from build123d import *

# Parameters (mm, degrees)
EXTRUDE1_DEPTH = 5.9944


with BuildPart() as part:
    # Sketch1 → Extrude1 (new body)
    with BuildSketch(Plane.XY):
        with BuildLine():
            Line((-209.059629258, -14.077865934), (-209.059629258, -29.477865934))
            Line((-209.059629258, -29.477865934), (58.656370742, -29.477865934))
            Line((58.656370742, -29.477865934), (58.656370742, -14.077865934))
            Line((58.656370742, -14.077865934), (64.650770742, -14.077865934))
            Line((64.650770742, -14.077865934), (64.650770742, -4.077865934))
            Line((64.650770742, -4.077865934), (58.656370742, -4.077865934))
            Line((58.656370742, -4.077865934), (58.656370742, 6.581535434))
            Line((58.656370742, 6.581535434), (49.512370742, 6.581535434))
            Line((49.512370742, 6.581535434), (49.512370742, 4.644785434))
            Line((49.512370742, 4.644785434), (45.512370742, 4.733384066))
            Line((45.512370742, 4.733384066), (45.512370742, 12.670884066))
            Line((45.512370742, 12.670884066), (49.512370742, 12.582285434))
            Line((49.512370742, 12.582285434), (49.512370742, 10.645535434))
            Line((49.512370742, 10.645535434), (58.656370742, 10.645535434))
            Line((58.656370742, 10.645535434), (58.656370742, 21.482134066))
            Line((58.656370742, 21.482134066), (64.650770742, 21.482134066))
            Line((64.650770742, 21.482134066), (64.650770742, 31.482134066))
            Line((64.650770742, 31.482134066), (58.656370742, 31.482134066))
            Line((58.656370742, 31.482134066), (58.656370742, 49.262134066))
            Line((58.656370742, 49.262134066), (27.756302278, 49.262134066))
            ThreePointArc((27.756302278, 49.262134066), (13.878151139, 27.724950493), (0, 49.262134066))
            Line((0, 49.262134066), (-209.059629258, 49.262134066))
            Line((-209.059629258, 49.262134066), (-209.059629258, 31.482134066))
            Line((-209.059629258, 31.482134066), (-215.054029258, 31.482134066))
            Line((-215.054029258, 31.482134066), (-215.054029258, 21.482134066))
            Line((-215.054029258, 21.482134066), (-209.059629258, 21.482134066))
            Line((-209.059629258, 21.482134066), (-209.059629258, 10.822732699))
            Line((-209.059629258, 10.822732699), (-199.915629258, 10.822732699))
            Line((-199.915629258, 10.822732699), (-199.915629258, 12.759482699))
            Line((-199.915629258, 12.759482699), (-195.915629258, 12.670884066))
            Line((-195.915629258, 12.670884066), (-195.915629258, 4.733384066))
            Line((-195.915629258, 4.733384066), (-199.915629258, 4.821982699))
            Line((-199.915629258, 4.821982699), (-199.915629258, 6.758732699))
            Line((-199.915629258, 6.758732699), (-209.059629258, 6.758732699))
            Line((-209.059629258, 6.758732699), (-209.059629258, -4.077865934))
            Line((-209.059629258, -4.077865934), (-215.054029258, -4.077865934))
            Line((-215.054029258, -4.077865934), (-215.054029258, -14.077865934))
            Line((-215.054029258, -14.077865934), (-209.059629258, -14.077865934))
        make_face()
    extrude(amount=EXTRUDE1_DEPTH)


solid = part.part
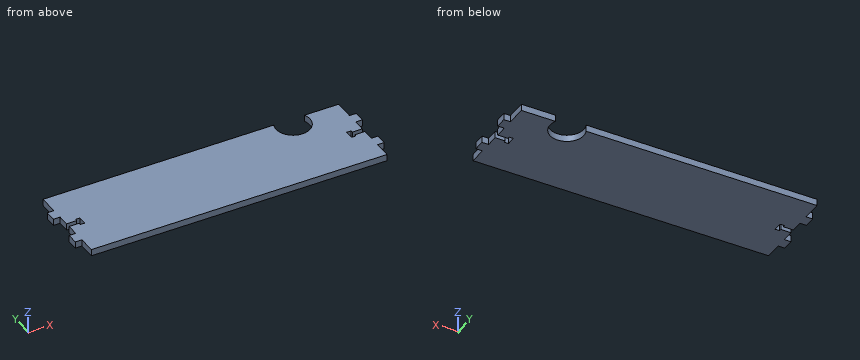
Work out the finished part from the listing and answer in its coordinate system (mm). Coordinates: 2 decimals unless noted, no trailing zeros. Loops run counter-clockwise (first coordinate to the right, second up) from the corner with the lowest first, then second, coordinate; pieces in that order, holes last. Notation, with made-up numbers: (65, 40.5) -> (114, 40.5) arc R30 ccw to (114, 65.5) -> close; hole circle Ø10 at (86, 80.5). An arc over 180 degrees is marked (long way). Write each question's results on one line, items separated by ' | '. Start each with the question number.
1) Consider line 1 along X through (y, z) = (-16, 4.4); line 2 along X through (y, z) = (39, 3.5); line 3 along X through (y, z) = (30, 2.7). Determine where each line is inside the solid, lowest interval first.
2) Find section C-C on x = 22. Determine the outline of the cut face in (y, z).
3) Find section B-B on y = -17.5. Determine the outline of the cut face in (x, z).
4) Find section A-A on y = 43. Determine the outline of the cut face in (x, z), then the cut area to 3 significant figures.
5) Flat-ended cylindrical pins translate along their axes: P1, Ø3, axis at y = 10.5, z = 3.5, coming from the -X side; P2, Ø1.8, axis at x = -212.5, z = 1.5, coming from the -Y side; P3, Ø1.5, axis at y = -17.5, z = 1.5, coming from the +X side. Find the tip coordinate at first contact, or state that the pin passes through.
Response values:
1) line 1: x = -209.06 to 58.66 | line 2: x = -209.06 to -0.84, 28.59 to 58.66 | line 3: x = -215.05 to 5.87, 21.89 to 64.65
2) outline: (-29.48, 0) -> (30.07, 0) -> (30.07, 5.99) -> (-29.48, 5.99) -> close
3) outline: (-209.06, 0) -> (58.66, 0) -> (58.66, 5.99) -> (-209.06, 5.99) -> close
4) outline: (-209.06, 0) -> (-1.36, 0) -> (-1.36, 5.99) -> (-209.06, 5.99) -> close; (29.12, 0) -> (58.66, 0) -> (58.66, 5.99) -> (29.12, 5.99) -> close | area: 1,420 mm^2
5) P1: stops at x = -209.06 | P2: stops at y = -14.08 | P3: stops at x = 58.66
